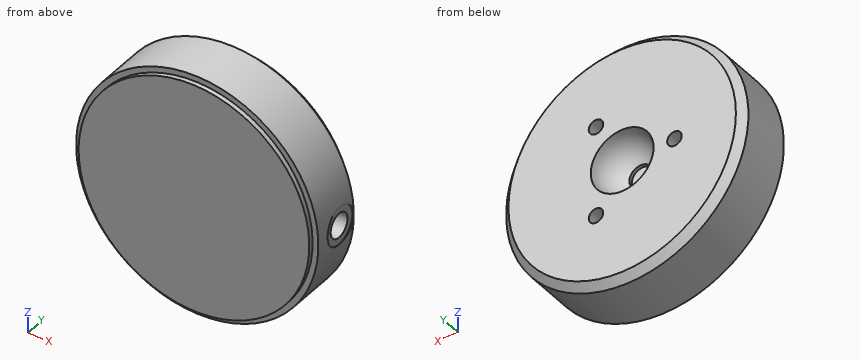
```python
from build123d import *

# Parameters (mm, degrees)
SKETCH1_R                          = 25
EXTRUDE1_DEPTH                     = 12.0142
CHAMFER1_SIZE                      = 1.524
F_3_16_0_1875_DIAMETER_HOLE1_D     = 4.7625
F_3_16_0_1875_DIAMETER_HOLE1_DEPTH = 6.2484
SKETCH5_R                          = 23.8062
EXTRUDE2_DEPTH                     = 0.98552
M5X0_8_TAPPED_HOLE1_D              = 4.2
M5X0_8_TAPPED_HOLE1_DEPTH          = 18.542
M5X0_8_TAPPED_HOLE1_CBORE_D        = 5
M5X0_8_TAPPED_HOLE1_CBORE_DEPTH    = 7.62
M5X0_8_TAPPED_HOLE1_TIP            = 1.2618073
CIRPATTERN1_COUNT                  = 3
SKETCH10_R                         = 3.937
CUT_EXTRUDE3_DEPTH                 = 0.381


with BuildPart() as part:
    # Sketch1 → Extrude1 (new body)
    with BuildSketch(Plane(origin=(0, 0, 0), x_dir=(1, 0, 0), z_dir=(0, 1, 0))):
        with Locations(Location((0, 0, 0), (0, 0, 270))):  # turned: the seam where the file's is
            Circle(SKETCH1_R)
    extrude(amount=EXTRUDE1_DEPTH)

    # Chamfer1
    chamfer1_edges = [part.edges().sort_by_distance(p)[0] for p in [
        (0, 12.0142, -25),
    ]]
    chamfer(chamfer1_edges, length=CHAMFER1_SIZE)

    # Sketch2 → Cut-Revolve1 (revolve, cut)
    with BuildSketch(Plane.XY):
        with BuildLine():
            Line((0, 19.0246), (0, 6.0198))
            ThreePointArc((0, 6.0198), (-6.5024, 12.5222), (0, 19.0246))
        make_face()
    revolve(axis=Axis((0, 19.0246, 0), (0, -1, 0)), mode=Mode.SUBTRACT)

    # 3_16 _0.1875_ Diameter Hole1
    with Locations(Plane(origin=(0, 12.0142, 0), x_dir=(-1, 0, 0), z_dir=(0, 1, 0))):
        with Locations((0, 0)):
            Hole(F_3_16_0_1875_DIAMETER_HOLE1_D / 2, depth=F_3_16_0_1875_DIAMETER_HOLE1_DEPTH)

    # Sketch5 → Extrude2 (add)
    with BuildSketch(Plane.XZ):
        with Locations(Location((0, 0, 0), (0, 0, 90))):  # turned: the seam where the file's is
            Circle(SKETCH5_R)
    extrude(amount=EXTRUDE2_DEPTH)

    # M5x0.8 Tapped Hole1
    with Locations(Plane(origin=(25, 6.6802, 0), x_dir=(0, 0, 1), z_dir=(1, 0, 0))):
        with Locations((0, 0)):
            CounterBoreHole(M5X0_8_TAPPED_HOLE1_D / 2, M5X0_8_TAPPED_HOLE1_CBORE_D / 2, M5X0_8_TAPPED_HOLE1_CBORE_DEPTH, depth=M5X0_8_TAPPED_HOLE1_DEPTH)
            with Locations((0, 0, -(M5X0_8_TAPPED_HOLE1_DEPTH + M5X0_8_TAPPED_HOLE1_TIP / 2))):  # 118° drill point
                Cone(0, M5X0_8_TAPPED_HOLE1_D / 2, M5X0_8_TAPPED_HOLE1_TIP, mode=Mode.SUBTRACT)

    # Sketch8 → M3x0.5 Tapped Hole1 (revolve, cut)
    with BuildSketch(Plane(origin=(-10.795, 12.0142, 0), x_dir=(0, 0, 1), z_dir=(1, 0, 0))):
        Polygon((0, 0), (0, 5.553072774), (1.25, 4.801997), (1.25, 3.302), (1.5, 3.302), (1.5, 0), align=None)
    m3x0_5_tapped_hole1 = revolve(axis=Axis((-10.795, 18.3642, 0), (0, -1, 0)), mode=Mode.SUBTRACT)

    # CirPattern1: M3x0.5 Tapped Hole1 ×3 about axis
    cirpattern1_axis = Axis((0, 0, 0), (0, 1, 0))
    for i in range(1, CIRPATTERN1_COUNT):
        add(m3x0_5_tapped_hole1.rotate(cirpattern1_axis, i * 360 / CIRPATTERN1_COUNT), mode=Mode.SUBTRACT)

    # Sketch10 → Cut-Extrude3 (cut)
    with BuildSketch(Plane(origin=(25, 5.2451, 0), x_dir=(0, 0, 1), z_dir=(1, 0, 0))):
        with Locations(Location((0, -1.4351, 0), (0, 0, 180))):  # turned: the seam where the file's is
            Circle(SKETCH10_R)
    extrude(amount=-CUT_EXTRUDE3_DEPTH, mode=Mode.SUBTRACT)


solid = part.part
```
Geometry check sheet. Reference: the model listing, model coordinates, mm. Give positions to 0.01 mm unless a question says otherwise; leave off trailing zeros. Order: outer loops, then holes, each group sorted by start corner. A loop starts at its lowest first (then second) coordinate and runs counter-clockwise, first axis right, second up. Notation, with made-up numbers: (5.25, -16.5) - (41.25, -16.5) arc R24 ccw to (41.25, -4.5) - close; hole circle Ø1 at (73.5, 86.25). An arc over 180 degrees is marked (long way). Write item = value, one per line. Start each with the question number.
1) Gauge pin test, flat ends, axial feed: pin 1 Ø3.5 at (y, z) = (6.68, 0) entering from -X; pin 2 Ø1.5 at (y, z) = (6, 11.5) entering from -X; pin 3 Ø0.9 at (x, z) = (6, -10) entering from +Y. Record the tip position at first contact, or that the pin passes through.
2) Section check A-A (x = 0). Enter the section's corners in (y, z).
3) Scan lines: L1, parallel to Z at x = 0, y = 6; L2, parallel to X at y = 11.05, z = 0 (3 decimals); L3, parallel to X at y = 8, z = 0 (3 decimals). Record each from-to range of solid material in increasing order.
4) Section check B-B (y = 8). Count the separate pieces of the cut face and the enclosed holes in it, then the cut area to 3 significant figures.
Geometry check:
q1.pin_1 = -25
q1.pin_2 = -22.57
q1.pin_3 = 8.71
q2.outline = (-0.99, -23.81) - (0, -23.81) - (0, -25) - (10.49, -25) - (12.01, -23.48) - (12.01, -6.48) arc R6.5 cw to (6.47, -2.38) - (5.77, -2.38) - (5.77, 2.38) - (6.47, 2.38) arc R6.5 cw to (12.01, 6.48) - (12.01, 23.48) - (10.49, 25) - (0, 25) - (0, 23.81) - (-0.99, 23.81) - close
q3.L1 = -25 to -2.38, 2.38 to 25
q3.L2 = -24.44 to -12.295, -9.295 to -6.334, 6.334 to 24.44
q3.L3 = -25 to -12.045, -9.545 to -4.672, 4.672 to 5.989
q4.separate_pieces = 1
q4.enclosed_holes = 4
q4.area = 1,810 mm2
